Drawing for the job (mm, zero at the part's lowest x, y, z). Round coordinates to 2 decimals unless told otherwise and drop trailing zeros. Order: outer loops, then holes, each group sorted by start corner. A loop starts at its lowest first (then second) coordinate and runs counter-clockwise, first axis right, second up. Notation, with made-up numbers: (53.25, 35.25) -> (74.25, 35.25) arc R23 ccw to (74.25, 53.25) -> close; hole circle Ø4 at (-28.5, 27). An arc over 180 degrees is marked (long way). Use CSV: the item, a comma, the result in double quotes.
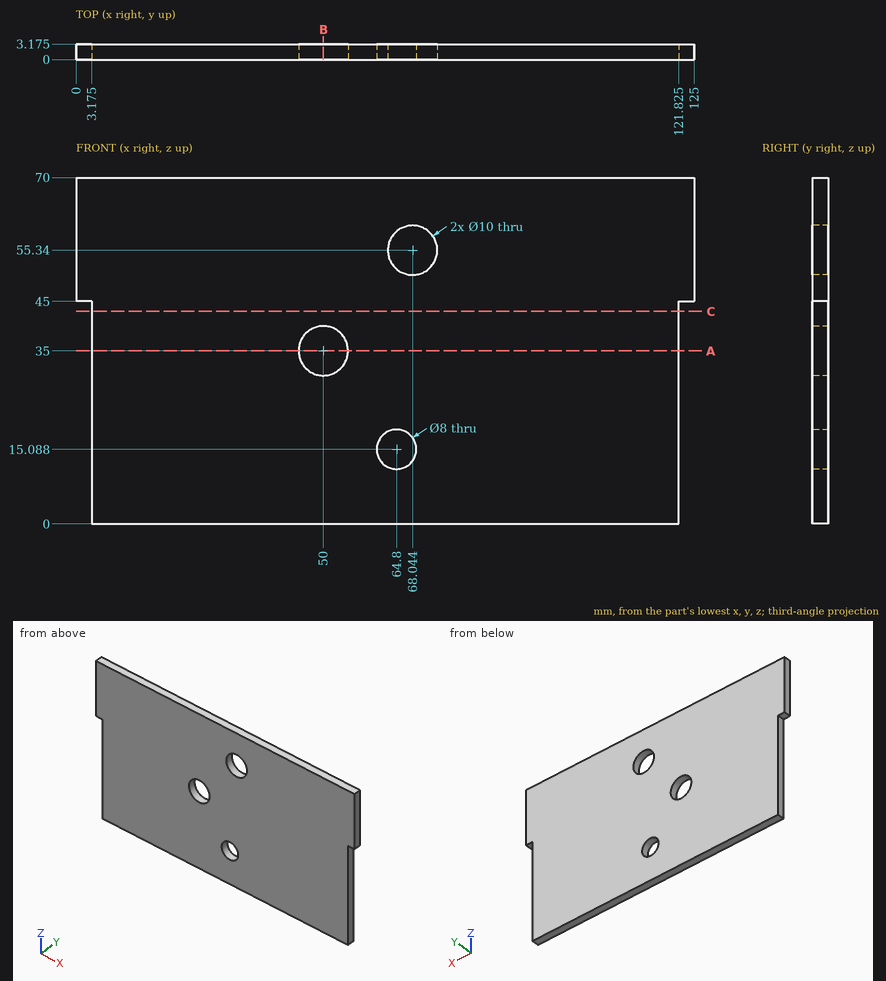
Q1. Cut at A-A (z = 35). Give the cut face in (x, y) (3 decimals).
From the geometry:
outline,"(3.175, 0) -> (45, 0) -> (45, 3.175) -> (3.175, 3.175) -> close; (55, 0) -> (121.825, 0) -> (121.825, 3.175) -> (55, 3.175) -> close"
Q2. Probe line 1 along Z through (x, y) = (50, 2.6); line 2 along X through (y, z) = (2, 55.5); line 3 along X through (y, z) = (2.45, 35) (3 decimals). List the from-to ranges inside material, lowest first.
From the geometry:
line 1,"z = 0 to 30, 40 to 70"
line 2,"x = 0 to 63.05, 73.04 to 125"
line 3,"x = 3.175 to 45, 55 to 121.825"
Q3. Cut at C-C (z = 43). Give the cut face in (x, y) (3 decimals), plus the area to 3 significant figures.
From the geometry:
outline,"(3.175, 0) -> (121.825, 0) -> (121.825, 3.175) -> (3.175, 3.175) -> close"
area,"377 mm²"
Q4. Pin check, flat tips, straight feed: pin 1 (1.6 mm diameter, centred on y = 2, z = 17, fed in from +X) (3 decimals); pin 2 (1.6 mm diameter, centred on x = 123.5, y = 1, fed in from -Z); pin 3 (1 mm diameter, centred on y = 1, z = 33.5, fed in from -X) (3 decimals). Stop position of each tip, or through.
From the geometry:
pin 1,"stops at x = 121.825"
pin 2,"stops at z = 45"
pin 3,"stops at x = 3.175"
Q5. Cut at B-B (x = 50). Give the cut face in (y, z) (3 decimals).
From the geometry:
outline,"(0, 0) -> (3.175, 0) -> (3.175, 30) -> (0, 30) -> close; (0, 40) -> (3.175, 40) -> (3.175, 70) -> (0, 70) -> close"
